Work out the finished part from the listing and answer in its coordinate system (mm). Face numbers are marked on the shaded views. A direction names the side the tool comes from. Coordinates: 2 decimals unless noted, no trailing zeros. Order: outer loops, then holes, each group sorted by start corner. A loop starts at its lowest first (then second) coordinate and runs counter-clockwise, first axis right, second up. Notation, with made-up numbers: M -5,47 L 30,47 A21 ccw 30,59 Z; hole C -20,80.25 d1. An arc over 180 degrees is marked long. Use a Markdown table: item, result. Add a question column.
from build123d import *

# Parameters (mm, degrees)
SKETCH_2_R          = 22.5
EXTRUDE_1_DEPTH     = 20
CUT_EXTRUDE_START   = -1
SKETCH_3_R          = 8.5
SKETCH_3_R_2        = 8
CUT_EXTRUDE_1_DEPTH = 1
EXTRUDE_2_DEPTH     = 20
HOLE_WIZARD_M31_D   = 2.5
CUT_EXTRUDE_2_DEPTH = 54.62107794515138
SKETCH_9_R          = 9.5
EXTRUDE_4_DEPTH     = 19
CUT_EXTRUDE_3_DEPTH = 18
SKETCH_14_R         = 8.000000000000538
CUT_EXTRUDE_5_DEPTH = 20.999999999999996
CUT_EXTRUDE_START_2 = -20.999999999999996
SKETCH_15_R         = 8
CUT_EXTRUDE_6_DEPTH = 20.999999999999996
SKETCH_13_R         = 8.5
SKETCH_13_R_2       = 8.000000000000538
CUT_EXTRUDE_7_DEPTH = 1


with BuildPart() as part:
    # Эскиз1 → Повернуть1 (revolve)
    with BuildSketch(Plane.XY, mode=Mode.PRIVATE) as revolve_1_sk:
        Polygon((6.000000000000004, 9.500000000000005), (6.0000000000000036, 10.500000000000005), (12.000000000000004, 9.500000000000005), (12.000000000000004, 10.500000000000005), (18.000000000000004, 9.500000000000009), (18.000000000000004, 10.500000000000005), (24.238502938920437, 9.460249510179933), (24.238502938920437, 10.460249510179935), (30, 9.50000000000001), (30, 10.750000000000004), (35.99999999999999, 9.250000000000005), (35.99999999999999, 8.000000000000004), (0, 8), (0, 9.500000000000005), align=None)
    revolve(revolve_1_sk.sketch.rotate(Axis((0, 0, 0), (1, 0, 0)), 90), axis=Axis((0, 0, 0), (1, 0, 0)))

    # Эскиз2 → Бобышка-Вытянуть1 (add)
    with BuildSketch(Plane.ZY):
        Circle(SKETCH_2_R)
    extrude(amount=EXTRUDE_1_DEPTH)

    # Эскиз3 → Вырез-Вытянуть1 (cut)
    with BuildSketch(Plane(origin=(35.99999999999999, 0, 0), x_dir=(0, 0, -1), z_dir=(1, 0, 0)).offset(CUT_EXTRUDE_START)):
        Circle(SKETCH_3_R)
        with Locations(Location((0, 0, 0), (0, 0, 180))):
            Circle(SKETCH_3_R_2, mode=Mode.SUBTRACT)
    extrude(amount=CUT_EXTRUDE_1_DEPTH, mode=Mode.SUBTRACT)

    # Эскиз4 → Бобышка-Вытянуть2 (add)
    with BuildSketch(Plane(origin=(0, 0, 0), x_dir=(0, 0, -1), z_dir=(1, 0, 0))):
        with BuildLine():
            Line((25.30000000000001, 2.799999999999917), (22.325097984107497, 2.7999999999999274))
            ThreePointArc((22.325097984107497, 2.7999999999999274), (22.500000000000007, -7.244e-14), (22.32509798410748, -2.8000000000000718))
            Line((22.32509798410748, -2.8000000000000718), (25.29999999999999, -2.8000000000000824))
            ThreePointArc((25.29999999999999, -2.8000000000000824), (28.099999999999998, -9.585e-14), (25.30000000000001, 2.799999999999917))
        make_face()
        with BuildLine():
            Line((-2.800000000000002, 25.3), (-2.800000000000002, 22.325097984107487))
            ThreePointArc((-2.800000000000002, 22.325097984107487), (1.38e-15, 22.500000000000007), (2.799999999999997, 22.32509798410749))
            Line((2.799999999999997, 22.32509798410749), (2.799999999999997, 25.3))
            ThreePointArc((2.799999999999997, 25.3), (5.9e-16, 28.099999999999998), (-2.800000000000002, 25.3))
        make_face()
        with BuildLine():
            Line((2.7999999999998266, -25.300000000000022), (2.7999999999998475, -22.325097984107504))
            ThreePointArc((2.7999999999998475, -22.325097984107504), (-1.535e-13, -22.500000000000004), (-2.800000000000152, -22.32509798410747))
            Line((-2.800000000000152, -22.32509798410747), (-2.800000000000173, -25.29999999999998))
            ThreePointArc((-2.800000000000173, -25.29999999999998), (-1.9663e-13, -28.099999999999998), (2.7999999999998266, -25.300000000000022))
        make_face()
        with BuildLine():
            Line((-25.300000000000026, -2.7999999999997374), (-22.32509798410751, -2.7999999999997685))
            ThreePointArc((-22.32509798410751, -2.7999999999997685), (-22.500000000000007, 2.3257e-13), (-22.32509798410746, 2.800000000000231))
            Line((-22.32509798410746, 2.800000000000231), (-25.299999999999972, 2.8000000000002623))
            ThreePointArc((-25.299999999999972, 2.8000000000002623), (-28.099999999999998, 2.9312e-13), (-25.300000000000026, -2.7999999999997374))
        make_face()
    extrude(amount=-EXTRUDE_2_DEPTH)

    # Отверстие обработанное метчиком M31 (through all)
    with Locations(Plane(origin=(0, 0, 0), x_dir=(0, 0, -1), z_dir=(1, 0, 0))):
        with Locations((0, 25.3), (-25.3, 0), (0, -25.3), (25.3, 0)):
            Hole(HOLE_WIZARD_M31_D / 2)

    # Эскиз7 → Вырез-Вытянуть2 (cut, through all)
    with BuildSketch(Plane(origin=(0, 0, 0), x_dir=(0, 0, -1), z_dir=(1, 0, 0))):
        with BuildLine():
            ThreePointArc((-22.32509798410751, -2.7999999999997685), (-14.424368200146956, -14.424368200146706), (-2.8000000000001526, -22.32509798410747))
            ThreePointArc((-2.8000000000001526, -22.32509798410747), (-15.90990257669746, -15.909902576697181), (-22.32509798410751, -2.7999999999997685))
        make_face()
    extrude(amount=-CUT_EXTRUDE_2_DEPTH, mode=Mode.SUBTRACT)

    # Эскиз9 → Бобышка-Вытянуть4 (add)
    with BuildSketch(Plane(origin=(0, -1.1520122757155562, 6.533386275242313), x_dir=(1, 0, 0), z_dir=(0, -0.17364817766692384, 0.9848077530122092))):
        with Locations(Location((-10.000000000000002, -11.99971468403886, 0), (0, 0, 270))):
            Circle(SKETCH_9_R)
    extrude(amount=EXTRUDE_4_DEPTH)

    # Эскиз10 → Повернуть2 (revolve)
    with BuildSketch(Plane(origin=(-10, 0, 0), x_dir=(0, 0, -1), z_dir=(1, 0, 0)), mode=Mode.PRIVATE) as revolve_2_sk:
        Polygon((-27.24654564763845, -27.65111017879284), (-27.4201938253054, -26.66630242578063), (-21.337699129565245, -26.609221112791218), (-21.771819573732436, -24.147201730261234), (-49.34643665807445, -29.009350704935), (-49.1293764359908, -30.240360396200256), (-44.92967315744145, -31.022979315050762), (-45.146733379525074, -29.79196962378552), (-39.3060208272686, -29.737157320947013), (-39.4796690049355, -28.752349567934818), (-33.155392165711675, -28.692999244794482), (-33.32904034337858, -27.70819149178227), align=None)
    revolve(revolve_2_sk.sketch.rotate(Axis((-10, -16.268739706163032, 23.161004995067916), (0, -0.1736481776669369, 0.9848077530122069)), 180), axis=Axis((-10, -16.268739706163032, 23.161004995067916), (0, -0.1736481776669369, 0.9848077530122069)))

    # Эскиз12 → Вырез-Вытянуть3 (cut)
    with BuildSketch(Plane.ZY.offset(20)):
        with BuildLine():
            ThreePointArc((20.373939602323045, -2.2699306334980194), (-14.495689014324347, 14.495689014324102), (2.2699306334983786, -20.37393960232301))
            ThreePointArc((2.2699306334983786, -20.37393960232301), (13.01015463777385, -13.01015463777362), (20.373939602323045, -2.2699306334980194))
        make_face()
    extrude(amount=-CUT_EXTRUDE_3_DEPTH, mode=Mode.SUBTRACT)

    # Эскиз14 → Вырез-Вытянуть5 (cut)
    with BuildSketch(Plane(origin=(0, -4.451327651387111, 25.244733582474296), x_dir=(1, 0, 0), z_dir=(0, -0.17364817766692386, 0.9848077530122094))):
        with Locations(Location((-10, -11.999714684038862, 0), (0, 0, 90))):
            Circle(SKETCH_14_R)
    extrude(amount=-CUT_EXTRUDE_5_DEPTH, mode=Mode.SUBTRACT)

    # Эскиз15 → Вырез-Вытянуть6 (cut)
    with BuildSketch(Plane(origin=(0, 0, 0), x_dir=(0, 0, -1), z_dir=(1, 0, 0)).offset(CUT_EXTRUDE_START_2)):
        with Locations(Location((0, 0, 0), (0, 0, 180))):
            Circle(SKETCH_15_R)
    extrude(amount=CUT_EXTRUDE_6_DEPTH, mode=Mode.SUBTRACT)

    # Эскиз13 → Вырез-Вытянуть7 (cut)
    with BuildSketch(Plane(origin=(0, -9.313476626061751, 52.81935066681644), x_dir=(1, 0, 0), z_dir=(0, -0.17364817766693696, 0.9848077530122069))):
        with Locations(Location((-10, -11.999714684038523, 0), (0, 0, 270))):
            Circle(SKETCH_13_R)
        with Locations(Location((-10, -11.999714684038523, 0), (0, 0, 7.531e-06))):
            Circle(SKETCH_13_R_2, mode=Mode.SUBTRACT)
    extrude(amount=-CUT_EXTRUDE_7_DEPTH, mode=Mode.SUBTRACT)


solid = part.part
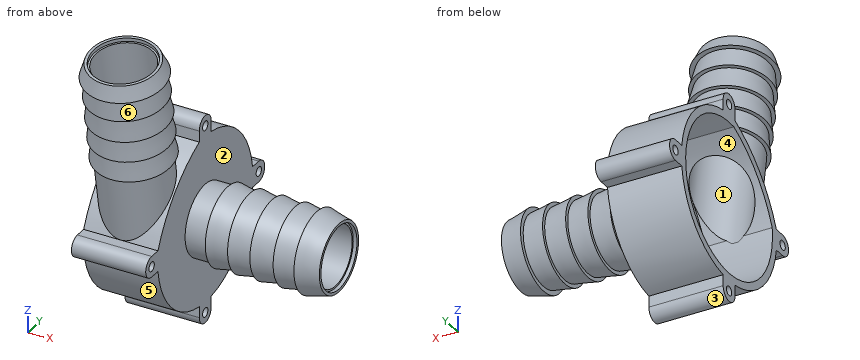
(1) A cutting plane is placed at D-D on y = 16.5. Write down the section's boundary in (x, z).
(2) A cutting plane is placed at B-B on x = 8. Write down the section's boundary in (y, z), plus the area to 3 significant figures.
(3) Given P1, Ø5, axis at x = -6.5, z = 31, coming from the -Y side; P2, Ø17, axis at y = -2, z = 1, coming from the -X side; P3, Ø2.5, axis at x = -14, y = 24, coming from the +Z side, each flat-ended and moving along its own axis, determine where each tip first touches the part or whether it passes through.
(4) A cutting plane is placed at C-C on z = -12. Write down the section's boundary in (x, y), plus the area to 3 significant figures.
(5) A cutting plane is placed at A-A on z = 0. Count the separate pieces of the cut face and the enclosed holes in it, plus the area to 3 significant figures.
(6) The mould has two halves that part along Y. Classify the marked faces 1, 2 and 3: pulls with the +Y half, pulls with the -Y half, needs draft (parallel to the pull), parting line crosses it, or undercut.
(7) Which of the six approach directions +Z, -Z, +X, -X, +Y, -Y give full straight-line access (tool end or side, diameter ignored) to the marked faces 4, 5 and 6?
(8) Straight lines are drawn through the part: line 1 (Y direction, x = -14.25, z = 0); line 2 (Y direction, x = 5, z = 0); line 3 (X direction, y = 1.5, z = -21.5). For each, find the intervals that lie inside material, in ascending order.
From the geometry:
| question | item | result |
|---|---|---|
| 1 | outline | M -20,-15.3 L 0,-15.3 L 0,15.3 L -20,15.3 L -20,12.17 L -2,12.17 L -2,-12.17 L -20,-12.17 Z |
| 2 | outline | C 0,0 d20.33; hole C 0,0 d16 |
| 2 | area | 124 mm2 |
| 3 | P1 | stops at y = -28.44 |
| 3 | P2 | stops at x = -2 |
| 3 | P3 | stops at z = 2.8 |
| 4 | outline | M -20,-19.03 L 0,-19.03 L 0,19.03 L -20,19.03 L -20,16.62 L -2,16.62 L -2,-16.62 L -20,-16.62 Z |
| 4 | area | 163 mm2 |
| 5 | separate pieces | 4 |
| 5 | enclosed holes | 0 |
| 5 | area | 391 mm2 |
| 6 | face 1 | undercut |
| 6 | face 2 | needs draft |
| 6 | face 3 | parting line crosses it |
| 7 | face 4 | -X |
| 7 | face 5 | -Z, +X, -X, -Y |
| 7 | face 6 | none |
| 8 | line 1 | y = -28.1 to -26.55, -24.05 to -20.5, 20.5 to 24.05, 26.55 to 28.1 |
| 8 | line 2 | y = -9.5 to -8, 8 to 9.5 |
| 8 | line 3 | x = -20 to 0 |
